Design review of the part built by this model. Coordinates are the model's own, in mm. Face numbers are marked on the shaded views. Coordinates: 2 decimals unless noted, no trailing zeros. Loops run counter-clockwise (first coordinate to the right, second up) from the corner with the lowest first, then second, coordinate; pieces in that order, holes last.
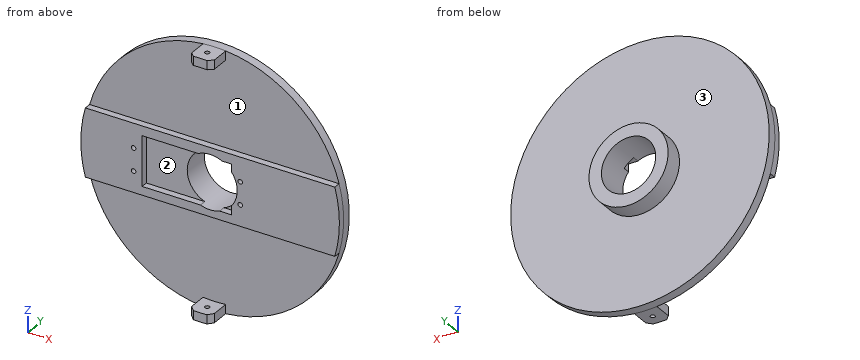
from build123d import *
from build123d.topology import SkipClean

# Parameters (mm, degrees)
SKETCH2_R               = 17.5
BOSS_EXTRUDE3_DEPTH     = 8
CUT_EXTRUDE3_DEPTH      = 8
CUT_EXTRUDE3_DEPTH_BACK = 10
SKETCH10_R              = 12
SKETCH11_W              = 54.5
SKETCH11_H              = 30
BOSS_EXTRUDE7_DEPTH     = 7
SKETCH12_W              = 39.5
SKETCH12_H              = 22
CUT_EXTRUDE4_DEPTH      = 43.148546831
SKETCH18_R              = 65
CUT_EXTRUDE6_DEPTH      = 4
SKETCH24_R              = 1
CUT_EXTRUDE7_DEPTH      = 4
SKETCH33_R              = 57.15
BOSS_EXTRUDE8_DEPTH     = 4
SKETCH34_R              = 12
CUT_EXTRUDE8_DEPTH      = 7
BOSS_EXTRUDE13_DEPTH    = 10
F_1_0MM_DOWEL_HOLE1_D   = 2
BOSS_EXTRUDE14_DEPTH    = 3
BOSS_EXTRUDE15_REACH    = 96.659
SKETCH21_W              = 30
SKETCH21_H              = 3
BOSS_EXTRUDE16_REACH    = 113.448
SKETCH31_W              = 30
SKETCH31_H              = 3
CHAMFER1_SIZE           = 2


with BuildPart() as part:
    # Sketch2 → Boss-Extrude3 (new body)
    with BuildSketch(Plane(origin=(0, 0, 0), x_dir=(1, 0, 0), z_dir=(0, 1, 0))):
        with Locations(Location((0, 0, 0), (0, 0, 270))):
            Circle(SKETCH2_R)
    extrude(amount=BOSS_EXTRUDE3_DEPTH)

    # Sketch10 → Cut-Extrude3 (cut, two sides: drawn at the far end of the back side and taken through both)
    with BuildSketch(Plane(origin=(0, 0, 0), x_dir=(1, 0, 0), z_dir=(0, 1, 0)).offset(-CUT_EXTRUDE3_DEPTH_BACK)):
        with Locations(Location((0, 0, 0), (0, 0, 270))):
            Circle(SKETCH10_R)
    extrude(amount=CUT_EXTRUDE3_DEPTH + CUT_EXTRUDE3_DEPTH_BACK, mode=Mode.SUBTRACT)

    # Sketch11 → Boss-Extrude7 (add)
    with BuildSketch(Plane(origin=(0, 0, 0), x_dir=(1, 0, 0), z_dir=(0, 1, 0))):
        with Locations((-10.25, 0)):
            Rectangle(SKETCH11_W, SKETCH11_H)
    extrude(amount=-BOSS_EXTRUDE7_DEPTH)

    # Sketch12 → Cut-Extrude4 (cut, through all)
    with BuildSketch(Plane(origin=(0, 0, 0), x_dir=(1, 0, 0), z_dir=(0, 1, 0))):
        with Locations((-10.311158619, 0.223490858)):
            Rectangle(SKETCH12_W, SKETCH12_H)
    extrude(amount=-CUT_EXTRUDE4_DEPTH, mode=Mode.SUBTRACT)

    # Sketch18 → Cut-Extrude6 (cut)
    with BuildSketch(Plane(origin=(0, 0, 0), x_dir=(1, 0, 0), z_dir=(0, 1, 0))):
        Circle(SKETCH18_R)
    extrude(amount=-CUT_EXTRUDE6_DEPTH, mode=Mode.SUBTRACT)


with BuildPart() as cut_extrude6_piece_1:
    # of the separate pieces the step leaves, piece 1, a body of its own (cut_extrude6_pieces)
    add(part.part.solids().sort_by_distance((0, 0, 17.5))[0])



with BuildPart() as cut_extrude6_piece_2:
    # of the separate pieces the step leaves, piece 2, a body of its own (cut_extrude6_pieces)
    add(part.part.solids().sort_by_distance((-37.5, -4, 15))[0])

    # Sketch24 → Cut-Extrude7 (cut)
    with BuildSketch(Plane.XZ.offset(7)):
        with Locations(Location((-33.811158619, 4.276509142, 0), (0, 0, 270))):
            Circle(SKETCH24_R)
        with Locations(Location((-33.811158619, -5.723490858, 0), (0, 0, 270))):
            Circle(SKETCH24_R)
        with Locations(Location((13.311158619, -5.723490858, 0), (0, 0, 90))):
            Circle(SKETCH24_R)
        with Locations(Location((13.311158619, 4.276509142, 0), (0, 0, 90))):
            Circle(SKETCH24_R)
    extrude(amount=-CUT_EXTRUDE7_DEPTH, mode=Mode.SUBTRACT)


with BuildPart() as cut_extrude6_piece_1_1:
    add(cut_extrude6_piece_1.part)

    add(cut_extrude6_piece_2.part)  # Boss-Extrude8 merges Cut-Extrude6 piece 2
    # Sketch33 → Boss-Extrude8 (add)
    with BuildSketch(Plane(origin=(0, 0, 0), x_dir=(1, 0, 0), z_dir=(0, 1, 0))):
        with Locations(Location((0, 0, 0), (0, 0, 270))):
            Circle(SKETCH33_R)
    extrude(amount=-BOSS_EXTRUDE8_DEPTH)

    # Sketch34 → Cut-Extrude8 (cut)
    with BuildSketch(Plane(origin=(0, 0, 0), x_dir=(1, 0, 0), z_dir=(0, 1, 0))):
        with Locations(Location((0, 0, 0), (0, 0, 270))):
            Circle(SKETCH34_R)
    extrude(amount=-CUT_EXTRUDE8_DEPTH, mode=Mode.SUBTRACT)

    # Sketch37 → Boss-Extrude13 (add)
    with SkipClean():  # the faces are left unmerged after this step: merging them gives an invalid solid
        with BuildSketch(Plane.XZ.offset(4)):
            with BuildLine():
                Line((-5, -52.91429391), (-5, -56.930857187))
                ThreePointArc((-5, -56.930857187), (0, -57.15), (5, -56.930857187))
                Line((5, -56.930857187), (5, -52.91429391))
                ThreePointArc((5, -52.91429391), (0, -53.15), (-5, -52.91429391))
            make_face()
            with BuildLine():
                Line((-5, 56.930857187), (-5, 52.91429391))
                ThreePointArc((-5, 52.91429391), (0, 53.15), (5, 52.91429391))
                Line((5, 52.91429391), (5, 56.930857187))
                ThreePointArc((5, 56.930857187), (0, 57.15), (-5, 56.930857187))
            make_face()
        extrude(amount=BOSS_EXTRUDE13_DEPTH)

    # Ø1.0mm Dowel Hole1 (through all)
    with Locations(Plane(origin=(0, -9, -57.15), x_dir=(-1, 0, 0), z_dir=(0, 0, -1))):
        with Locations((0, 0)):
            Hole(F_1_0MM_DOWEL_HOLE1_D / 2)

    # Sketch86 → Boss-Extrude14 (add)
    with SkipClean():  # the faces are left unmerged after this step: merging them gives an invalid solid
        with BuildSketch(Plane(origin=(0, -4, 0), x_dir=(-1, 0, 0), z_dir=(0, -1, 0))):
            with BuildLine():
                Line((-51.119442268, -15), (-55.146373408, -15))
                ThreePointArc((-55.146373408, -15), (-57.15, 0), (-55.146373408, 15))
                Line((-55.146373408, 15), (-51.119442268, 15))
                ThreePointArc((-51.119442268, 15), (-53.274734892, 0), (-51.119442268, -15))
            make_face()
            with BuildLine():
                Line((51.119442268, -15), (55.146373408, -15))
                ThreePointArc((55.146373408, -15), (57.15, 0), (55.146373408, 15))
                Line((55.146373408, 15), (51.119442268, 15))
                ThreePointArc((51.119442268, 15), (53.274734892, 0), (51.119442268, -15))
            make_face()
        extrude(amount=BOSS_EXTRUDE14_DEPTH)

    # Sketch21 → Boss-Extrude15 (add, up to next)
    with BuildSketch(Plane(origin=(17, 0, 0), x_dir=(0, 0, -1), z_dir=(1, 0, 0)), mode=Mode.PRIVATE) as boss_extrude15_sk1:
        with Locations((0, -5.5)):
            Rectangle(SKETCH21_W, SKETCH21_H)
    boss_extrude15_tool1 = extrude(boss_extrude15_sk1.sketch, amount=BOSS_EXTRUDE15_REACH, mode=Mode.PRIVATE) - cut_extrude6_piece_1_1.part
    add(boss_extrude15_tool1.solids().sort_by_distance((17, -5.5, 0))[0])

    # Sketch31 → Boss-Extrude16 (add, up to next)
    with BuildSketch(Plane.ZY.offset(37.5), mode=Mode.PRIVATE) as boss_extrude16_sk1:
        with Locations((0, -5.5)):
            Rectangle(SKETCH31_W, SKETCH31_H)
    boss_extrude16_tool1 = extrude(boss_extrude16_sk1.sketch, amount=BOSS_EXTRUDE16_REACH, mode=Mode.PRIVATE) - cut_extrude6_piece_1_1.part
    add(boss_extrude16_tool1.solids().sort_by_distance((-37.5, -5.5, 0))[0])

    # Chamfer1
    chamfer1_edges = [cut_extrude6_piece_1_1.edges().sort_by_distance(p)[0] for p in [
        (5, -14, -54.922575548),
        (-5, -14, -54.922575548),
        (-5, -14, 54.922575548),
        (5, -14, 54.922575548),
    ]]
    chamfer(chamfer1_edges, length=CHAMFER1_SIZE)


solid = cut_extrude6_piece_1_1.part
Q1. The part is to be moulded in two halves that separate along Z. For the marked faces 1, 2 and 3, say which applies: pulls with the +Z half, pulls with the -Z half, needs draft (parallel to the pull), parting line crosses it, or undercut.
Q2. Take a section at A-A, the plane z = 0. Write out the cut boundary in (x, y), then the cut area to 3 significant figures.
Q3. Take a section at D-D, the plane x = -26. Write out the cut boundary in (y, z), then the cut area to 3 significant figures.
Q4. Take a section at C-C, the plane y = 2.5. Write out the cut boundary in (x, z), then the cut area to 3 significant figures.
Q5. For line 1 (X direction, y = -9, z = 55.9); line 2 (X direction, y = 0.25, z = 0); line 3 (Y direction, x = -6, z = 22), list the stretches that pass through material, from the lowest coordinate up.
Q6. Clearance check with flat-ended pins moving along their axes: pin 1 Ø1.8 at (x, z) = (-33.81, 4.28) entering from +Y; pin 2 Ø6 at (x, y) = (-27, 2) entering from -Z; pin 3 Ø0.9 at (y, z) = (-6, -10) entering from -X; pin 4 Ø2.5 at (x, y) = (0, -9) entering from -Z. State where each tip first meets the part, or that it passes through.
Q7. Take a section at B-B, the plane x = -8. Write out the cut boundary in (y, z), then the cut area to 3 significant figures.
Entries:
1. face 1: undercut
1. face 2: undercut
1. face 3: needs draft
2. outline: (-57.15, -7) - (-30.06, -7) - (-30.06, -4) - (-12, -4) - (-12, 8) - (-17.5, 8) - (-17.5, 0) - (-57.15, 0) - close; (12, -7) - (57.15, -7) - (57.15, 0) - (17.5, 0) - (17.5, 8) - (12, 8) - close
2. area: 666 mm2
3. outline: (-7, -15) - (-4, -15) - (-4, -50.89) - (0, -50.89) - (0, 50.89) - (-4, 50.89) - (-4, 15) - (-7, 15) - (-7, 10.78) - (-4, 10.78) - (-4, -11.22) - (-7, -11.22) - close
3. area: 431 mm2
4. outline: circle Ø35 at (0, 0); hole circle Ø24 at (0, 0)
4. area: 510 mm2
5. line 1: x = -5 to -1, 1 to 5
5. line 2: x = -17.5 to -12, 12 to 17.5
5. line 3: y = -4 to 0
6. pin 1: stops at y = 0
6. pin 2: stops at z = -51.51
6. pin 3: stops at x = -56.35
6. pin 4: stops at z = -57.15
7. outline: (-7, -15) - (-4, -15) - (-4, -56.59) - (0, -56.59) - (0, -15.56) - (8, -15.56) - (8, -8.94) - (-4, -8.94) - (-4, -11.22) - (-7, -11.22) - close; (-7, 10.78) - (-4, 10.78) - (-4, 8.94) - (8, 8.94) - (8, 15.56) - (0, 15.56) - (0, 56.59) - (-4, 56.59) - (-4, 15) - (-7, 15) - close
7. area: 511 mm2
